Drawing for the job (mm, zero at the part's lowest x, y, z). A direction names the side the tool comes from. Give positions to 0.01 mm unless a question says otherwise; leave off trailing zeros. Write each loop counter-clockwise with the first axis right and the second up, starting at its lowest first coordinate (ties: lowest second). Pieces come first, ordered by that corner, then holes.
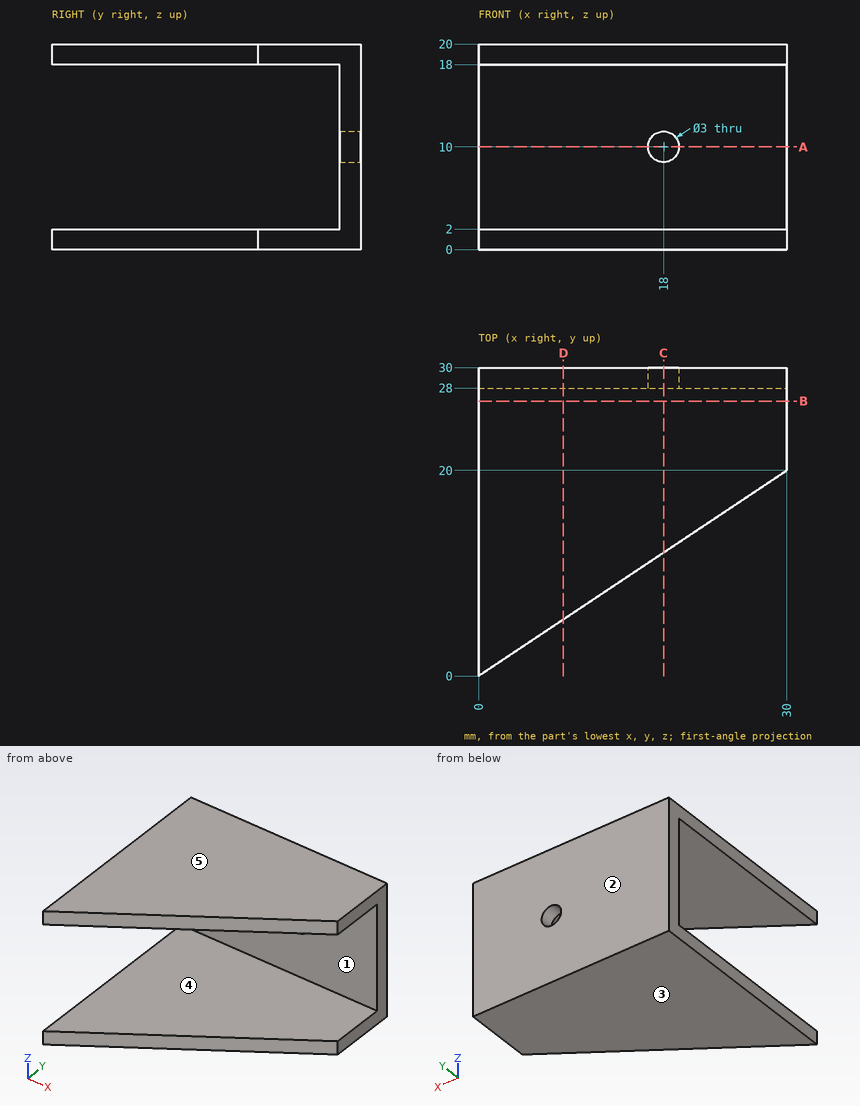
1. Which spindle directions (+Z, -Z, +X, -X, +Y, -Y) get a long thin tool onto all of the face, cutting with end or side? Do the marked faces 4 and 5. Say none if no direction does.
Calculated:
face 4: +X, -X, -Y
face 5: +Z, +X, -X, +Y, -Y
2. Slice it at C-C, the plane x = 18. Write the cut outline in (y, z).
Calculated:
outline: (12, 0) - (30, 0) - (30, 8.5) - (28, 8.5) - (28, 2) - (12, 2) - close; (12, 18) - (28, 18) - (28, 11.5) - (30, 11.5) - (30, 20) - (12, 20) - close
3. Slice it at B-B, the plane y = 26.75. Write the cut outline in (x, z).
Calculated:
outline: (0, 0) - (30, 0) - (30, 2) - (0, 2) - close; (0, 18) - (30, 18) - (30, 20) - (0, 20) - close
4. Slice it at A-A, the plane z = 10. Write the cut outline in (x, y), and give its area (3 significant figures).
Calculated:
outline: (0, 28) - (16.5, 28) - (16.5, 30) - (0, 30) - close; (19.5, 28) - (30, 28) - (30, 30) - (19.5, 30) - close
area: 54.0 mm2
5. Pull direction Z, two halves, no side cores. Call the marked faces 1, 2 and 3: +Z half, -Z half, draft (parallel to the pull), parting line (faces both ways), or undercut.
Calculated:
face 1: undercut
face 2: draft
face 3: -Z half
6. Pin check, flat tips, straight feed: P1, Ø12, axis at y = 14, z = 12.5, coming from the -X side; P2, Ø5, axis at x = 12, z = 7, coming from the -Y side. Stop position of each tip, or through.
Calculated:
P1: stops at x = 0
P2: stops at y = 28
7. Probe probe 1 along Z at (x, y) = (14, 9.5); probe 2 along X at (y, z) = (29.05, 10); probe 3 along Z at (x, y) = (18, 29). List the from-to ranges inside material, lowest first.
Calculated:
probe 1: z = 0 to 2, 18 to 20
probe 2: x = 0 to 16.5, 19.5 to 30
probe 3: z = 0 to 8.5, 11.5 to 20
8. Slice it at D-D, the plane x = 8.25. Write the cut outline in (y, z).
Calculated:
outline: (5.5, 0) - (30, 0) - (30, 20) - (5.5, 20) - (5.5, 18) - (28, 18) - (28, 2) - (5.5, 2) - close
